from build123d import *

# Parameters (mm, degrees)
SKETCH1_W           = 1000
SKETCH1_H           = 500
SKETCH1_W_2         = 996
SKETCH1_H_2         = 496
EXTRUDE_THIN1_DEPTH = 500
SKETCH2_W           = 500
SKETCH2_H           = 1000
SKETCH2_W_2         = 496
SKETCH2_H_2         = 996
EXTRUDE_THIN2_DEPTH = 250
CUT_EXTRUDE1_REACH  = 752
SKETCH3_W           = 496
SKETCH3_H           = 996


with BuildPart() as part:
    # Sketch1 → Extrude-Thin1 (new body, symmetric)
    with BuildSketch(Plane(origin=(0, 0, 0), x_dir=(0, 0, -1), z_dir=(1, 0, 0))):
        Rectangle(SKETCH1_W, SKETCH1_H)
        Rectangle(SKETCH1_W_2, SKETCH1_H_2, mode=Mode.SUBTRACT)
    extrude(amount=EXTRUDE_THIN1_DEPTH, both=True)

    # Sketch2 → Extrude-Thin2 (add)
    with BuildSketch(Plane.XZ.offset(250)):
        Rectangle(SKETCH2_W, SKETCH2_H)
        Rectangle(SKETCH2_W_2, SKETCH2_H_2, mode=Mode.SUBTRACT)
    extrude(amount=EXTRUDE_THIN2_DEPTH)

    # Sketch3 → Cut-Extrude1 (cut, up to next)
    with BuildSketch(Plane.XZ.offset(500), mode=Mode.PRIVATE) as cut_extrude1_sk1:
        Rectangle(SKETCH3_W, SKETCH3_H)
    cut_extrude1_tool1 = extrude(cut_extrude1_sk1.sketch, amount=-CUT_EXTRUDE1_REACH, mode=Mode.PRIVATE) & part.part
    add(cut_extrude1_tool1.solids().sort_by_distance((0, -500, 0))[0], mode=Mode.SUBTRACT)


solid = part.part
Work out the finished part from the listing and answer in its coordinate system (mm). A direction names the side the tool comes from. Coordinates: 2 decimals unless noted, no trailing zeros. Loops run counter-clockwise (first coordinate to the right, second up) from the corner with the lowest first, then second, coordinate; pieces in that order, holes last. Notation, with made-up numbers: (88.5, 7) -> (132.5, 7) arc R15 ccw to (132.5, 13) -> close; hole circle Ø7 at (-8.75, 27.5). An arc over 180 degrees is marked (long way). Write each question's results on one line, items separated by ' | '. Start each with the question number.
1) For faces 1 (the flat face through (7, -48, -498)), 2 (the flat face through (248, -372, -7)), 3 (the flat face through (377, -250, 7)), 4 (the flat face through (-373, -250, 7)), determine the directions among +Z, -Z, +X, -X, +Y, -Y from which every point of the face is accessible in a straight line to the end or side of a thin tool.
2) The mould has two halves that part along X. Classify faces 5 (the flat face through (-372, -248, 7)), 6 (the flat face through (250, -373, -7)), 7 (the flat face through (-248, -372, -7)), 8 (the flat face through (7, -48, 498)): pulls with the +X half, pulls with the -X half, needs draft (parallel to the pull), parting line crosses it, or undercut.
3) Find section C-C on z = -243. Determine the outline of the cut face in (x, y), then the cut area to 3 significant figures.
4) Consider line 1 along X through (y, z) = (-313, 454.5); line 2 along Z through (x, y) = (452.5, -235). Determine where each line is inside the solid, lowest interval first.
5) Find section B-B on x = 437.5. Determine the outline of the cut face in (y, z), then the cut area to 3 significant figures.
6) Flat-ended cylindrical pins translate along their axes: P1, Ø3, axis at x = 326.5, z = 124.5, coming from the -Y side; P2, Ø1, axis at y = -299.5, z = 235.5, coming from the -X side. Find the tip coordinate at first contact, or state that the pin passes through.
7) Find section A-A on y = -180.5. Determine the outline of the cut face in (x, z).
Response values:
1) face 1: none | face 2: -Y | face 3: +Z, -Z, +X, -Y | face 4: +Z, -Z, -X, -Y
2) face 5: needs draft | face 6: pulls with the +X half | face 7: undercut | face 8: undercut
3) outline: (-500, -250) -> (-250, -250) -> (-250, -500) -> (-248, -500) -> (-248, -248) -> (-500, -248) -> close; (-500, 248) -> (500, 248) -> (500, 250) -> (-500, 250) -> close; (248, -500) -> (250, -500) -> (250, -250) -> (500, -250) -> (500, -248) -> (248, -248) -> close | area: 4,010 mm^2
4) line 1: x = -250 to -248, 248 to 250 | line 2: z = -500 to -498, 498 to 500
5) outline: (-250, -500) -> (250, -500) -> (250, 500) -> (-250, 500) -> close; hole (-248, -498) -> (248, -498) -> (248, 498) -> (-248, 498) -> close | area: 5,980 mm^2
6) P1: stops at y = -250 | P2: stops at x = -250
7) outline: (-500, -500) -> (500, -500) -> (500, -498) -> (-500, -498) -> close; (-500, 498) -> (500, 498) -> (500, 500) -> (-500, 500) -> close
